Build history of the part. All positions in model axes, mm. Face numbers are marked on the shaded views. Round coordinates to 2 decimals unless told otherwise and drop trailing zeros. Write each loop counter-clockwise with the first axis right and the second up, starting at its lowest first coordinate (ties: lowest second). Pieces come first, ordered by that corner, then holes.
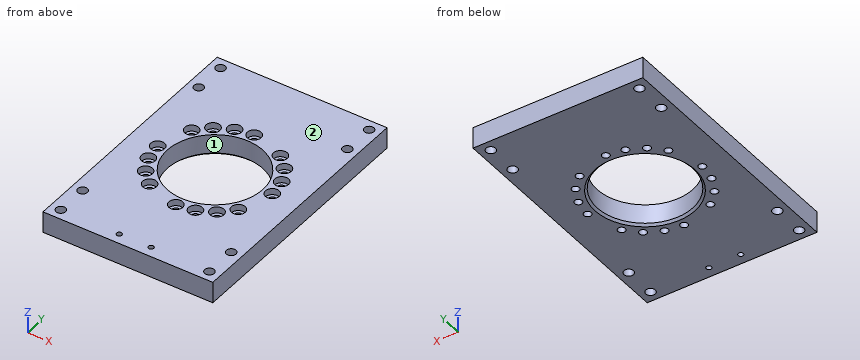
from build123d import *

# Parameters (mm, degrees)
SKETCH1_W                                           = 80
SKETCH1_H                                           = 120
SKETCH1_R                                           = 22.5
BOSS_EXTRUDE1_DEPTH                                 = 10
CBORE_FOR_M3_HEX_SOCKET_HEAD_CAP_SCREW1_D           = 3.5
CBORE_FOR_M3_HEX_SOCKET_HEAD_CAP_SCREW1_CBORE_D     = 6.5
CBORE_FOR_M3_HEX_SOCKET_HEAD_CAP_SCREW1_CBORE_DEPTH = 3
CHAMFER1_SIZE                                       = 1
F_4_5_4_5_DIAMETER_HOLE1_D                          = 4.5
M3_TAPPED_HOLE1_D                                   = 2.5


with BuildPart() as part:
    # Sketch1 → Boss-Extrude1 (new body)
    with BuildSketch(Plane.XY):
        Rectangle(SKETCH1_W, SKETCH1_H)
        Circle(SKETCH1_R, mode=Mode.SUBTRACT)
    extrude(amount=BOSS_EXTRUDE1_DEPTH)

    # CBORE for M3 Hex Socket Head Cap Screw1 (through all)
    with Locations(Plane.XY.offset(10)):
        with Locations((-27, 0), (-25.67852594, -8.343458848), (-21.843458848, -15.870201812), (-15.870201812, -21.843458848), (27, 0), (25.67852594, 8.343458848), (21.843458848, 15.870201812), (15.870201812, 21.843458848), (0, 27), (-8.343458848, 25.67852594), (-15.870201812, 21.843458848), (-21.843458848, 15.870201812), (0, -27), (8.343458848, -25.67852594), (15.870201812, -21.843458848), (21.843458848, -15.870201812)):
            CounterBoreHole(CBORE_FOR_M3_HEX_SOCKET_HEAD_CAP_SCREW1_D / 2, CBORE_FOR_M3_HEX_SOCKET_HEAD_CAP_SCREW1_CBORE_D / 2, CBORE_FOR_M3_HEX_SOCKET_HEAD_CAP_SCREW1_CBORE_DEPTH)

    # Chamfer1
    chamfer1_edges = [part.edges().sort_by_distance(p)[0] for p in [
        (-22.5, 0, 0),
    ]]
    chamfer(chamfer1_edges, length=CHAMFER1_SIZE)

    # Ø4.5 (4.5) Diameter Hole1 (through all)
    with Locations(Plane.XY.offset(10)):
        with Locations((-35, 55), (35, 55), (35, -55), (-35, -55), (-35, -40), (-35, 40), (35, 40), (35, -40)):
            Hole(F_4_5_4_5_DIAMETER_HOLE1_D / 2)

    # M3 Tapped Hole1 (through all)
    with Locations(Plane(origin=(0, 0, 0), x_dir=(-1, 0, 0), z_dir=(0, 0, -1))):
        with Locations((-7.5, -55), (7.5, -55)):
            Hole(M3_TAPPED_HOLE1_D / 2)


solid = part.part
1) Mould opens along X. For the marked faces 1 and 2 say: released by +X, released by -X, zero draft, split by the parting line, or undercut.
Results:
face 1: undercut
face 2: zero draft
2) Slice it at D-D (z = 8.75). Count the separate pieces of the cut face and the enclosed holes in it, plus the area to 3 significant figures.
Results:
separate pieces: 1
enclosed holes: 27
area: 7,340 mm2
3) Slice it at C-C (y = 40). Write the cut outline in (x, z), plus the area to 3 significant figures.
Results:
outline: (-40, 0) - (-37.25, 0) - (-37.25, 10) - (-40, 10) - close; (-32.75, 0) - (32.75, 0) - (32.75, 10) - (-32.75, 10) - close; (37.25, 0) - (40, 0) - (40, 10) - (37.25, 10) - close
area: 710 mm2
4) Slice it at B-B (x = 0). Write the cut outline in (y, z).
Results:
outline: (-60, 0) - (-28.75, 0) - (-28.75, 7) - (-30.25, 7) - (-30.25, 10) - (-60, 10) - close; (-25.25, 0) - (-23.5, 0) - (-22.5, 1) - (-22.5, 10) - (-23.75, 10) - (-23.75, 7) - (-25.25, 7) - close; (22.5, 1) - (23.5, 0) - (25.25, 0) - (25.25, 7) - (23.75, 7) - (23.75, 10) - (22.5, 10) - close; (28.75, 0) - (60, 0) - (60, 10) - (30.25, 10) - (30.25, 7) - (28.75, 7) - close
5) Slice it at A-A (y = -55). Write the cut outline in (x, z), plus the area to 3 significant figures.
Results:
outline: (-40, 0) - (-37.25, 0) - (-37.25, 10) - (-40, 10) - close; (-32.75, 0) - (-8.75, 0) - (-8.75, 10) - (-32.75, 10) - close; (-6.25, 0) - (6.25, 0) - (6.25, 10) - (-6.25, 10) - close; (8.75, 0) - (32.75, 0) - (32.75, 10) - (8.75, 10) - close; (37.25, 0) - (40, 0) - (40, 10) - (37.25, 10) - close
area: 660 mm2
6) Pin check, flat tips, straight feed: pin 1 Ø2 at (x, y) = (-15.87, -21.84) entering from +Z; pin 2 Ø3 at (x, y) = (-14.5, -22) entering from +Z. Stop position of each tip, or through.
Results:
pin 1: passes through
pin 2: stops at z = 7
7) Wall check: L1, parallel to Y at x = 35, z = 6; L2, parallel to Y at x = 26, z = 9; L3, parallel to X at y = 15.5, z = 2.25. Give the ranges that are in metal, low to high.
Results:
L1: y = -60 to -57.25, -52.75 to -42.25, -37.75 to 37.75, 42.25 to 52.75, 57.25 to 60
L2: y = -60 to -3.09, 3.09 to 5.11, 11.58 to 60
L3: x = -40 to -23.55, -20.13 to -16.31, 16.31 to 20.13, 23.55 to 40
